Design review of the part built by this model. Coordinates are the model's own, in mm. A direction names the side the tool comes from. Coordinates: 2 decimals unless noted, no trailing zeros. Loops run counter-clockwise (first coordinate to the right, second up) from the corner with the lowest first, then second, coordinate; pieces in that order, holes last. Notation, with made-up numbers: M 89,46 L 107,46 A20 cw 107,53 Z; hole C -24.5,31.25 d1. An arc over 180 degrees is marked long. Answer as CSV lines item,"result". Start each with the question number.
from build123d import *

# Parameters (mm, degrees)
SKETCH_1_R          = 50
EXTRUDE_1_DEPTH     = 3
SKETCH_2_R          = 50
SKETCH_2_R_2        = 47
EXTRUDE_2_DEPTH     = 350
SKETCH_3_R          = 3
CUT_EXTRUDE_1_DEPTH = 350


with BuildPart() as part:
    # Эскиз1 → Бобышка-Вытянуть1 (new body)
    with BuildSketch(Plane.XY):
        Circle(SKETCH_1_R)
    extrude(amount=EXTRUDE_1_DEPTH)

    # Эскиз2 → Бобышка-Вытянуть2 (add)
    with BuildSketch(Plane.XY.offset(3)):
        Circle(SKETCH_2_R)
        Circle(SKETCH_2_R_2, mode=Mode.SUBTRACT)
    extrude(amount=EXTRUDE_2_DEPTH)

    # Эскиз3 → Вырез-Вытянуть1 (cut)
    with BuildSketch(Plane(origin=(0, 0, 0), x_dir=(-1, 0, 0), z_dir=(0, 0, -1))):
        Circle(SKETCH_3_R)
    extrude(amount=-CUT_EXTRUDE_1_DEPTH, mode=Mode.SUBTRACT)


solid = part.part
Item 1: Mouldability with a two-part tool opening along Y and no side actions: class faces 3 (the face through (-34, -33, 353)), 4 (the face through (47.69, 15.02, 174.03)), 5 (the face through (3, 0, 1)), 6 (the face through (-1, -10, 3)) as released by +Y, released by -Y, zero draft, split by the parting line, or undercut.
Item 2: For line 1 along Y through (x, z) = (0, 2); line 2 along Y through (x, z) = (0, 267); line 3 along Z through (x, y) = (26, -13), list the stretches that pass through material, from the lowest coordinate up. Write a range as from..to.
Item 3: Add section C-C (y = 19). Give the boundary of the cut face in (x, z), plus the area to 3 significant figures.
Item 4: For pin 1 (7 mm diameter, centred on x = 0, y = 0, fed in from +Z); pin 2 (10 mm diameter, centred on x = -20, z = 86, fed in from -Y); pin 3 (3 mm diameter, centred on x = 38, z = 83, fed in from -Y), all flat-tipped, find the tip position at first contact; note any pin that passes through.
Item 5: Add section B-B (x = 35). Give the boundary of the cut face in (y, z), plus the area to 3 significant figures.
Item 6: Add section A-A (z = 46). Give the boundary of the cut face in (x, y).
Item 7: For faces 1 (the face through (-1, -10, 0)), 2 (the face through (44.83, 14.12, 175.55)), list the 3-axis set-ups (+Z, -Z, +X, -X, +Y, -Y) from which the entire face can be reached by the end or side of a thin tool; tool diameter is ignored.
Response:
1,face 3,"zero draft"
1,face 4,"split by the parting line"
1,face 5,"undercut"
1,face 6,"undercut"
2,line 1,"-50..-3, 3..50"
2,line 2,"-50..-47, 47..50"
2,line 3,"0..3"
3,outline,"M -46.25,0 L 46.25,0 L 46.25,353 L 42.99,353 L 42.99,3 L -42.99,3 L -42.99,353 L -46.25,353 Z"
3,area,"2,560 mm²"
4,pin 1,"z = 3"
4,pin 2,"y = -47.7"
4,pin 3,"y = -34.17"
5,outline,"M -35.71,0 L 35.71,0 L 35.71,353 L 31.37,353 L 31.37,3 L -31.37,3 L -31.37,353 L -35.71,353 Z"
5,area,"3,250 mm²"
6,outline,"C 0,0 d100; hole C 0,0 d94"
7,face 1,"-Z, +X, -X, +Y, -Y"
7,face 2,"+Z"
